Autodesk Inventor part; units mm, degrees
ref_plane "Work Plane1" through (0, 0, 127) normal (0, 0, 1) x (1, 0, 0)
ref_plane "YZ Plane" through (0, 0, 0) normal (1, 0, 0) x (0, 1, 0)
ref_plane "XZ Plane" through (0, 0, 0) normal (0, 1, 0) x (-1, 0, 0)
sketch "Sketch1" plane through (0, 0, 0) normal (0, 0, 1) x (1, 0, 0)
  line L0 (2.1997, 3.81) -> (4.3994, 0)
  line L1 (4.3994, 0) -> (2.1997, -3.81)
  line L2 (2.1997, -3.81) -> (-2.1997, -3.81)
  line L3 (-2.1997, -3.81) -> (-4.3994, 0)
  line L4 (-4.3994, 0) -> (-2.1997, 3.81)
  line L5 (-2.1997, 3.81) -> (2.1997, 3.81)
  line L6 (0, 0) -> (1.0543, 0)
  dimension "d0" = 7.62
extrude "Extrusion1" add sketch "Sketch1" along normal blind 228.6
ref_plane "Work Plane1" through (0, 0, 127) normal (0, 0, 1) x (1, 0, 0)
sketch "Sketch2" plane through (0, 0, 127) normal (0, 0, 1) x (1, 0, 0)
  line L0 (2.1997, 3.81) -> (4.3994, 0) construction
  line L1 (4.3994, 0) -> (2.1997, -3.81)
  line L2 (2.1997, -3.81) -> (-2.1997, -3.81)
  line L3 (-2.1997, -3.81) -> (-4.3994, 0)
  line L4 (-4.3994, 0) -> (-2.1997, 3.81)
  line L5 (-2.1997, 3.81) -> (2.1997, 3.81)
  circle A0 centre (0, 0) radius 25.4
  circle A1 centre (0, 0) radius 20.32
  circle A2 centre (0, 0) radius 10.795
  line L6 (-2.1997, 3.81) -> (-4.3994, 0)
  line L7 (-4.3994, 0) -> (-2.1997, -3.81)
  line L8 (2.1997, -3.81) -> (4.3994, 0)
  line L9 (2.1997, 3.81) -> (-2.1997, 3.81)
  line L10 (4.3994, 0) -> (2.1997, 3.81)
  line L11 (-4.3994, 0) -> (-20.32, 0)
  line L12 (4.3994, 0) -> (20.32, 0)
  line L13 (10.4919, -2.54) -> (20.1606, -2.54)
  line L14 (10.4919, 2.54) -> (20.1606, 2.54)
  line L15 (-10.4919, 2.54) -> (-20.1606, 2.54)
  line L16 (-10.4919, -2.54) -> (-20.1606, -2.54)
  line L17 (-2.1997, 3.81) -> (-10.16, 17.5976)
  line L18 (2.1997, 3.81) -> (10.16, 17.5976)
  line L19 (-2.1997, -3.81) -> (2.1997, -3.81)
  line L20 (2.1997, -3.81) -> (10.16, -17.5976)
  line L21 (-2.1997, -3.81) -> (-10.16, -17.5976)
  line L22 (-7.4457, 7.8163) -> (-12.28, 16.1896)
  line L23 (-3.0463, 10.3563) -> (-7.8806, 18.7296)
  line L24 (3.0463, 10.3563) -> (7.8806, 18.7296)
  line L25 (7.4457, 7.8163) -> (12.28, 16.1896)
  line L26 (7.4457, -7.8163) -> (12.28, -16.1896)
  line L27 (3.0463, -10.3563) -> (7.8806, -18.7296)
  line L28 (-7.4457, -7.8163) -> (-12.28, -16.1896)
  line L29 (-3.0463, -10.3563) -> (-7.8806, -18.7296)
  dimension "d6" = 21.59
  dimension "d4" = 50.8
  dimension "d5" = 5.08
  dimension "d31" = 5.08
  dimension "d32" = 2.54
  dimension "d33" = 5.08
  dimension "d34" = 2.54
  dimension "d35" = 120
  dimension "d36" = 120
  dimension "d37" = 120
  dimension "d38" = 120
  dimension "d39" = 5.08
  dimension "d40" = 2.54
  dimension "d41" = 5.08
  dimension "d42" = 2.54
  dimension "d44" = 5.08
  dimension "d45" = 2.54
  dimension "d46" = 5.08
  dimension "d47" = 2.54
extrude "Extrusion3" add sketch "Sketch2" along normal blind 12.7 contours L12 A2 L20 L1 | L10 L18 A2 L12 | L20 A2 L21 L2 | L5 L17 A2 L18 | L12 A1 L13 A2 | A2 L14 A1 L12 | L21 A2 L11 L3 | L20 A1 L27 A2 | A2 L26 A1 L20 | L4 L11 A2 L17 | L18 A1 L25 A2 | A2 L24 A1 L18 | L21 A1 L28 A2 | A2 L29 A1 L21 | L17 A1 L23 A2 | A2 L22 A1 L17 | L11 A1 L15 A2 | A2 L16 A1 L11 | A0
equation "\"d36\" = d35"
equation "\"d37\" = d35"
equation "\"d38\" = d35"
properties part number "RobotArm HexWheel"
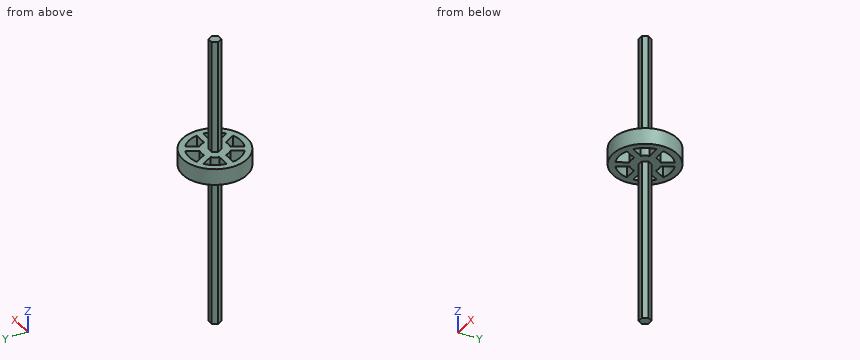
Work out the finished part from the listing and answer in its coordinate system (mm). Coordinates: 2 decimals unless noted, no trailing zeros. Loops run counter-clockwise (first coordinate to the right, second up) from the corner with the lowest first, then second, coordinate; pieces in that order, holes last. Notation, with made-up numbers: M 33.25,81.25 L 44.25,81.25 A27 ccw 44.25,118.25 Z; hole C -8.5,-20 d2. An arc over 180 degrees is marked long. Answer in a Markdown table with one row per item. Add a question column.
1. Find section B-B, the plane z = 56.5. Write down the section's boundary in (x, y).
2. Flat-ended cylindrical pins translate along their axes: P1, Ø10.5, axis at x = -16.5, z = 136, coming from the -Y side; P2, Ø3.5, axis at x = 1, z = 176.5, coming from the +Y side; P3, Ø3, axis at x = 0.5, y = 5.5, coming from the +Z side. Find the tip coordinate at first contact, or state that the pin passes through.
3. Find section A-A, the plane x = 0. Write down the section's boundary in (y, z) (3 decimals), then the cut area to 3 significant figures.
4. Find section C-C, the plane x = -14.5. Write down the section's boundary in (y, z).
5. Consider L1, parallel to Y at x = 1, z = 134; L2, parallel to Y at x = -17, z = 134; L3, parallel to X at y = 3.5, z = 127.5. Determine where each line is inside the solid, lowest interval first.
6. Find section D-D, the plane x = 15. Write down the section's boundary in (y, z).
Reported:
| question | item | result |
|---|---|---|
| 1 | outline | M -4.4,0 L -2.2,-3.81 L 2.2,-3.81 L 4.4,0 L 2.2,3.81 L -2.2,3.81 Z |
| 2 | P1 | stops at y = -22.77 |
| 2 | P2 | stops at y = 3.81 |
| 2 | P3 | stops at z = 139.7 |
| 3 | outline | M -25.4,127 L -20.32,127 L -20.32,139.7 L -25.4,139.7 Z; M -10.795,127 L -3.81,127 L -3.81,0 L 3.81,0 L 3.81,127 L 10.795,127 L 10.795,139.7 L 3.81,139.7 L 3.81,228.6 L -3.81,228.6 L -3.81,139.7 L -10.795,139.7 Z; M 20.32,127 L 25.4,127 L 25.4,139.7 L 20.32,139.7 Z |
| 3 | area | 2,050 mm^2 |
| 4 | outline | M -20.85,127 L -14.24,127 L -14.24,139.7 L -20.85,139.7 Z; M -2.54,127 L 2.54,127 L 2.54,139.7 L -2.54,139.7 Z; M 14.24,127 L 20.85,127 L 20.85,139.7 L 14.24,139.7 Z |
| 5 | L1 | y = -25.38 to -20.3, -10.75 to 10.75, 20.3 to 25.38 |
| 5 | L2 | y = -18.87 to -11.13, -2.54 to 2.54, 11.13 to 18.87 |
| 5 | L3 | x = -25.16 to -20.02, -10.21 to 10.21, 20.02 to 25.16 |
| 6 | outline | M -20.5,127 L -13.71,127 L -13.71,139.7 L -20.5,139.7 Z; M -2.54,127 L 2.54,127 L 2.54,139.7 L -2.54,139.7 Z; M 13.71,127 L 20.5,127 L 20.5,139.7 L 13.71,139.7 Z |
